Work out the finished part from the listing and answer in its coordinate system (mm). Face numbers are marked on the shaded views. A direction names the side the tool comes from. Round coordinates to 2 decimals unless told otherwise and drop trailing zeros. Loops run counter-clockwise (first coordinate to the right, second up) from the corner with the lowest first, then second, coordinate; pieces in that order, holes last. Notation, with made-up numbers: (55, 30.5) - (106, 30.5) arc R23 cw to (106, 51.5) - close; hole circle Ø5 at (33, 63.25). An arc over 180 degrees is marked (long way). Return JSON: item names as keys, results as strings.
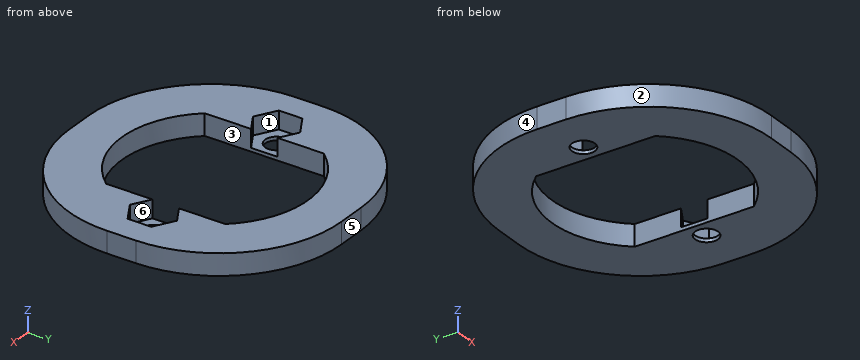
from build123d import *

# Parameters (mm, degrees)
BOSS_EXTRUDE5_DEPTH = 3
SKETCH2_R           = 1.6
CUT_EXTRUDE2_DEPTH  = 4
CUT_EXTRUDE3_DEPTH  = 2.5


with BuildPart() as part:
    # Sketch1 → Boss-Extrude5 (new body)
    with BuildSketch(Plane.XY):
        with BuildLine():
            Line((-1.997893001, -19), (1.997893001, -19))
            ThreePointArc((1.997893001, -19), (14.018708281, -14.02081528), (18.997893001, -2))
            Line((18.997893001, -2), (18.997893001, 2))
            ThreePointArc((18.997893001, 2), (14.018708281, 14.02081528), (1.997893001, 19))
            Line((1.997893001, 19), (-1.997893001, 19))
            ThreePointArc((-1.997893001, 19), (-14.018708281, 14.02081528), (-18.997893001, 2))
            Line((-18.997893001, 2), (-18.997893001, -2))
            ThreePointArc((-18.997893001, -2), (-14.018708281, -14.02081528), (-1.997893001, -19))
        make_face()
        with BuildLine():
            Line((-10, -8.306623863), (-10, 8.306623863))
            ThreePointArc((-10, 8.306623863), (0, 13), (10, 8.306623863))
            Line((10, 8.306623863), (10, -8.306623863))
            ThreePointArc((10, -8.306623863), (0, -13), (-10, -8.306623863))
        make_face(mode=Mode.SUBTRACT)
    extrude(amount=BOSS_EXTRUDE5_DEPTH)

    # Sketch2 → Cut-Extrude2 (cut, through all)
    with BuildSketch(Plane.XY.offset(3)):
        with Locations((-12.5, 0)):
            Circle(SKETCH2_R)
        with Locations((12.5, 0)):
            Circle(SKETCH2_R)
    extrude(amount=-CUT_EXTRUDE2_DEPTH, mode=Mode.SUBTRACT)

    # Sketch3 → Cut-Extrude3 (cut)
    with BuildSketch(Plane.XY.offset(3)):
        Polygon((-12.5, 3.290896534), (-15.35, 1.645448267), (-15.35, -1.645448267), (-12.5, -3.290896534), (-9.65, -1.645448267), (-9.65, 1.645448267), align=None)
        Polygon((12.5, 3.290896534), (9.65, 1.645448267), (9.65, -1.645448267), (12.5, -3.290896534), (15.35, -1.645448267), (15.35, 1.645448267), align=None)
    extrude(amount=-CUT_EXTRUDE3_DEPTH, mode=Mode.SUBTRACT)


solid = part.part
1) Determine the mould class of the marked faces 4, 5 and 6 for opening direction X: pulls with the +X half, pulls with the -X half, needs draft (parallel to the pull), parting line crosses it, or undercut.
Verdict:
{"face 4": "pulls with the -X half", "face 5": "needs draft", "face 6": "undercut"}
2) Section C-C (x = -3) is taken. Give the vertices of the cut face in (y, z), and give its area (3 significant figures).
Verdict:
{"outline": "(-18.97, 0) - (-12.65, 0) - (-12.65, 3) - (-18.97, 3) - close; (12.65, 0) - (18.97, 0) - (18.97, 3) - (12.65, 3) - close", "area": "37.9 mm2"}
3) Section A-A (y = 0) is taken. Give the vertices of the cut face in (x, z).
Verdict:
{"outline": "(-19, 0) - (-14.1, 0) - (-14.1, 0.5) - (-15.35, 0.5) - (-15.35, 3) - (-19, 3) - close; (-10.9, 0) - (-10, 0) - (-10, 0.5) - (-10.9, 0.5) - close; (10, 0) - (10.9, 0) - (10.9, 0.5) - (10, 0.5) - close; (14.1, 0) - (19, 0) - (19, 3) - (15.35, 3) - (15.35, 0.5) - (14.1, 0.5) - close"}
4) Find the intervals of material crossed by L1, parallel to X at y = 0.5, z = 2.55; L2, parallel to X at y = -8.5, z = 1.75; L3, parallel to Y at x = -12.5, z = 0.3, in increasing order.
Verdict:
{"L1": "x = -19 to -15.35, 15.35 to 19", "L2": "x = -17.71 to -9.84, 9.84 to 17.71", "L3": "y = -15.37 to -1.6, 1.6 to 15.37"}
5) A tool of negligible diameter and unlimited length cuts with its end or side. For the marked faces 1, 2 and 3, from which of +Z, -Z, +X, -X, +Y, -Y can it reach the whole face along a straight path? Write none if from no direction.
Verdict:
{"face 1": "+Z", "face 2": "+Z, -Z, -X, -Y", "face 3": "+Z, -Z"}
6) Flat-ended cylindrical pins translate along their axes: pin 1 (1.6 mm diameter, centred on x = 13.5, y = 1.5, fed in from +Z); pin 2 (1.5 mm diameter, centred on y = -9.5, z = 1, fed in from +X); pin 3 (2.5 mm diameter, centred on x = 12.5, y = 0, fed in from -Z); pin 4 (0.9 mm diameter, centred on y = 3.5, z = 1.5, fed in from +X). Find the tip coordinate at first contact, or state that the pin passes through.
Verdict:
{"pin 1": "stops at z = 0.5", "pin 2": "stops at x = 17.6", "pin 3": "passes through", "pin 4": "stops at x = 18.97"}
7) Section B-B (z = 1.3) is taken. Give the vertices of the cut face in (x, y), and give its area (3 significant figures).
Verdict:
{"outline": "(-19, -2) arc R17 ccw to (-2, -19) - (2, -19) arc R17 ccw to (19, -2) - (19, 2) arc R17 ccw to (2, 19) - (-2, 19) arc R17 ccw to (-19, 2) - close; hole (-15.35, -1.65) - (-12.5, -3.29) - (-10, -1.85) - (-10, -8.31) arc R13 ccw to (10, -8.31) - (10, -1.85) - (12.5, -3.29) - (15.35, -1.65) - (15.35, 1.65) - (12.5, 3.29) - (10, 1.85) - (10, 8.31) arc R13 ccw to (-10, 8.31) - (-10, 1.85) - (-12.5, 3.29) - (-15.35, 1.65) - close", "area": "679 mm2"}
8) Section D-D (y = 7) is taken. Give the vertices of the cut face in (x, z), and give its area (3 significant figures).
Verdict:
{"outline": "(-18.25, 0) - (-10, 0) - (-10, 3) - (-18.25, 3) - close; (10, 0) - (18.25, 0) - (18.25, 3) - (10, 3) - close", "area": "49.5 mm2"}
